from build123d import *

# Parameters (mm, degrees)
ESBO_O1_R                = 20.863274014
RESSALTO_EXTRUS_O1_DEPTH = 10


with BuildPart() as part:
    # Esboço1 → Ressalto-extrusão1 (new body)
    with BuildSketch(Plane.XY):
        with BuildLine():
            Line((7335.845216731, 5491.256809223), (7400.784408374, 5530.976897315))
            ThreePointArc((7400.784408374, 5530.976897315), (7413.321768246, 5536.451480894), (7426.873657559, 5538.323045473))
            Line((7426.873657559, 5538.323045473), (7573.061256946, 5538.323045473))
            ThreePointArc((7573.061256946, 5538.323045473), (7614.474439212, 5516.339974903), (7619.472065145, 5469.720978859))
            Line((7619.472065145, 5469.720978859), (7564.300408584, 5332.071693766))
            ThreePointArc((7564.300408584, 5332.071693766), (7561.033258012, 5307.80390458), (7569.680866385, 5284.894981989))
            Line((7569.680866385, 5284.894981989), (7662.336085762, 5151.851296041))
            ThreePointArc((7662.336085762, 5151.851296041), (7663.61020686, 5089.017265945), (7600.799568851, 5091.153261173))
            Line((7600.799568851, 5091.153261173), (7551.417263378, 5132.063170982))
            ThreePointArc((7551.417263378, 5132.063170982), (7536.472634142, 5140.597670031), (7519.519540605, 5143.559466201))
            Line((7519.519540605, 5143.559466201), (7393.552869473, 5143.559466201))
            ThreePointArc((7393.552869473, 5143.559466201), (7373.972219734, 5147.552964967), (7357.519382018, 5158.895539969))
            Line((7357.519382018, 5158.895539969), (7335.845216731, 5181.426044959))
            Line((7335.845216731, 5181.426044959), (7335.845216731, 5213.722321046))
            ThreePointArc((7335.845216731, 5213.722321046), (7353.706243942, 5339.368656723), (7338.756279232, 5465.394513266))
            ThreePointArc((7338.756279232, 5465.394513266), (7333.313540231, 5477.876860759), (7335.845216731, 5491.256809223))
        make_face()
        with Locations((7566.174846652, 5169.295330687)):
            Circle(ESBO_O1_R, mode=Mode.SUBTRACT)
        with Locations((7633.216444383, 5119.830887551)):
            Circle(ESBO_O1_R, mode=Mode.SUBTRACT)
        with Locations((7581.43197041, 5491.256809223)):
            Circle(ESBO_O1_R, mode=Mode.SUBTRACT)
        with BuildLine():
            Line((7512.734775832, 5486.974409199), (7433.320588265, 5486.974409199))
            ThreePointArc((7433.320588265, 5486.974409199), (7421.471766691, 5498.823230773), (7433.320588265, 5510.672052347))
            Line((7433.320588265, 5510.672052347), (7512.734775832, 5510.672052347))
            ThreePointArc((7512.734775832, 5510.672052347), (7521.55530344, 5498.823230773), (7512.734775832, 5486.974409199))
        make_face(mode=Mode.SUBTRACT)
        with BuildLine():
            Line((7530.423638246, 5301.620805578), (7451.009450679, 5301.620805578))
            ThreePointArc((7451.009450679, 5301.620805578), (7439.160629105, 5313.469627152), (7451.009450679, 5325.318448726))
            Line((7451.009450679, 5325.318448726), (7530.423638246, 5325.318448726))
            ThreePointArc((7530.423638246, 5325.318448726), (7539.244165855, 5313.469627152), (7530.423638246, 5301.620805578))
        make_face(mode=Mode.SUBTRACT)
    extrude(amount=RESSALTO_EXTRUS_O1_DEPTH)


solid = part.part
Can you work these out from the model? Positions are in its coordinate system, mm. A direction names the side the tool comes from. Coordinates: 2 decimals unless noted, no trailing zeros. Write each loop counter-clockwise with the first axis right and the second up, starting at its lowest first coordinate (ties: lowest second). Pieces come first, ordered by that corner, then holes. Notation, with made-up numbers: (60.5, 60) -> (86.5, 60) arc R26 ccw to (86.5, 77) -> close; hole circle Ø8 at (-3.75, 7). An arc over 180 degrees is marked (long way). Write each question's results on one line, items separated by ' | '. Start each with the question number.
Item 1: Please list where these lines run through material, in increasing order: probe 1 along Y at (x, z) = (7468, 9.75); probe 2 along Y at (x, z) = (7609, 9); probe 3 along X at (y, z) = (5156.5, 8).
Item 2: On a 3-axis mill with a long thin cutter (end or side, diameter ignored), from which of +Z, -Z, +X, -X, +Y, -Y can I reach the whole of each face in a straight line? I mean faces 4 (the flat face through (7576.454, 5111.322, 4.93)), 5 (the cylindrical face through (7439.163, 5313.209, 4.93)), 6 (the flat face through (7615.36, 5219.304, 4.93)). Say none if no direction works.
Item 3: If we section it at D-D, the plane z = 1.5: Write out the boundary of the cut face in (x, y).
Item 4: If we section it at B-B, the plane y = 5475: Write out the boundary of the cut face in (x, z), and give its area (3 significant figures).
Item 5: If we section it at C-C, the plane x = 7632: Write out the boundary of the cut face in (y, z), and give its area (3 significant figures).
Item 6: If we section it at A-A, the plane x = 7488.5: Write out the boundary of the cut face in (y, z), and give its area (3 significant figures).
Item 7: Thinking about a two-plate mould opening in Y: for faces 1 (the cylindrical face through (7664.303, 5089.717, 4.93)), 2 (the cylindrical face through (7333.336, 5477.685, 4.93)), 3 (the flat face through (7457, 5143.559, 5)), which applies, released by +Y, released by -Y, zero draft, split by the parting line, or undercut?
Item 8: I'm going to push flat-ended pins straight in: P1, Ø1.5, axis at x = 7494, z = 4.5, coming from the -Y side; P2, Ø4, axis at x = 7579, z = 8, coming from the +Y side; P3, Ø1, axis at x = 7616.5, z = 2.5, coming from the +Y side. Where does each tip first touch, or does it pass through?
Answer block:
1) probe 1: 5143.56 to 5301.62, 5325.32 to 5486.97, 5510.67 to 5538.32 | probe 2: 5083.96 to 5228.44, 5443.59 to 5523.09 | probe 3: 7359.99 to 7549.7, 7582.65 to 7659.1
2) face 4: +Z, -Z, -X, -Y | face 5: +Z, -Z | face 6: +Z, -Z, +X
3) outline: (7335.85, 5181.43) -> (7357.52, 5158.9) arc R50 ccw to (7393.55, 5143.56) -> (7519.52, 5143.56) arc R50 cw to (7551.42, 5132.06) -> (7600.8, 5091.15) arc R43.28 ccw (long way) to (7662.34, 5151.85) -> (7569.68, 5284.89) arc R50 cw to (7564.3, 5332.07) -> (7619.47, 5469.72) arc R50 ccw to (7573.06, 5538.32) -> (7426.87, 5538.32) arc R50 ccw to (7400.78, 5530.98) -> (7335.85, 5491.26) arc R23.11 ccw to (7338.76, 5465.39) arc R490.84 cw to (7335.85, 5213.72) -> close; hole (7433.32, 5486.97) -> (7512.73, 5486.97) arc R12.37 ccw to (7512.73, 5510.67) -> (7433.32, 5510.67) arc R11.85 ccw to start; hole (7451.01, 5301.62) -> (7530.42, 5301.62) arc R12.37 ccw to (7530.42, 5325.32) -> (7451.01, 5325.32) arc R11.85 ccw to start; hole circle Ø41.73 at (7566.17, 5169.3); hole circle Ø41.73 at (7581.43, 5491.26); hole circle Ø41.73 at (7633.22, 5119.83)
4) outline: (7333.82, 0) -> (7568.36, 0) -> (7568.36, 10) -> (7333.82, 10) -> close; (7594.51, 0) -> (7621.25, 0) -> (7621.25, 10) -> (7594.51, 10) -> close | area: 2,610 mm²
5) outline: (5076.57, 0) -> (5099, 0) -> (5099, 10) -> (5076.57, 10) -> close; (5140.66, 0) -> (5195.41, 0) -> (5195.41, 10) -> (5140.66, 10) -> close | area: 772 mm²
6) outline: (5143.56, 0) -> (5301.62, 0) -> (5301.62, 10) -> (5143.56, 10) -> close; (5325.32, 0) -> (5486.97, 0) -> (5486.97, 10) -> (5325.32, 10) -> close; (5510.67, 0) -> (5538.32, 0) -> (5538.32, 10) -> (5510.67, 10) -> close | area: 3,470 mm²
7) face 1: split by the parting line | face 2: undercut | face 3: released by -Y
8) P1: y = 5143.56 | P2: y = 5538.17 | P3: y = 5513.94
